Source: CAD feature listing. Evaluate the final solid. Frame: model axes, mm. A direction names the side the tool comes from. Coordinates: 2 decimals unless noted, no trailing zeros. Order: outer loops, then holes, each group sorted by start corner. A loop starts at its lowest first (then second) coordinate and runs counter-clockwise, first axis right, second up. Notation, with made-up numbers: (-14.5, 47) -> (16.5, 47) arc R10 ccw to (16.5, 66) -> close; hole circle Ø4 at (-38.75, -11.75). An arc over 180 degrees is marked (long way). Write item = value, one per line. Start each with the question number.
Item 1: Ray query, line 1 along Y through (x, z) = (0, 3.5); line 2 along X through (y, z) = (15, 4.25); line 3 along Y through (x, z) = (-2.5, 5.2). Return the intervals inside material, ascending. Write a range as [from, to].
Item 2: Set-up query: faces 5 (the flat face through (3, -33, 2)), 6 (the flat face through (0, 21, 3)), 7 (the flat face through (3, -33, 4)), 8 (the flat face through (-2, -33, 3)). Return all of +Z, -Z, +X, -X, +Y, -Y with unobstructed straight access to the full face (end or side cutting, diameter ignored); none if empty.
Item 3: Contact query for flat-ended pins moving along their axis: pin 1 (4.5 mm diameter, centred on x = 0.5, y = -34, fed in from +Z); pin 2 (2 mm diameter, centred on x = -6, z = 3, fed in from -Y); pin 3 (3.5 mm diameter, centred on y = -34.5, z = 2.5, fed in from -X). Output: stop coordinate, or through.
Item 4: Section query A-A (x = -6.75). Output: boundary loops of the cut face in (y, z).
Item 5: Section query D-D (x = 0). Output: boundary loops of the cut face in (y, z).
Item 6: Section query C-C (z = 3.1). Output: boundary loops of the cut face in (x, y), then the cut area to 3 significant figures.
Item 7: Mould query, pull axis Y, two halves, no side actions, for faces 1 (the flat face through (0, -31.8, 1.5)), 2 (the flat face through (0, -21, 3)), 3 (the flat face through (0, 28, 3)), 4 (the flat face through (-10, 0, 3)). Classes: released by +Y, released by -Y, zero draft, split by the parting line, or undercut.
Item 8: Section query B-B (y = -33). Output: boundary loops of the cut face in (x, z), then the cut area to 3 significant figures.
```python
from build123d import *

# Parameters (mm, degrees)
SKETCH1_W           = 28
SKETCH1_H           = 56
SKETCH1_W_2         = 20
SKETCH1_H_2         = 42
BOSS_EXTRUDE1_DEPTH = 6
SKETCH2_W           = 4
SKETCH2_H           = 3
SKETCH2_W_2         = 1.5
SKETCH2_H_2         = 2
BOSS_EXTRUDE2_DEPTH = 10
SKETCH3_R           = 1
CUT_EXTRUDE1_DEPTH  = 10


with BuildPart() as part:
    # Sketch1 → Boss-Extrude1 (new body)
    with BuildSketch(Plane.XY):
        Rectangle(SKETCH1_W, SKETCH1_H)
        Rectangle(SKETCH1_W_2, SKETCH1_H_2, mode=Mode.SUBTRACT)
    extrude(amount=BOSS_EXTRUDE1_DEPTH)

    # Sketch2 → Boss-Extrude2 (add)
    with BuildSketch(Plane.XZ.offset(28)):
        with Locations((0, 3)):
            Rectangle(SKETCH2_W, SKETCH2_H)
        with Locations((2.75, 3)):
            Rectangle(SKETCH2_W_2, SKETCH2_H_2)
    extrude(amount=BOSS_EXTRUDE2_DEPTH)

    # Sketch3 → Cut-Extrude1 (cut)
    with BuildSketch(Plane.XY.offset(4.5)):
        with Locations((0, -33)):
            Circle(SKETCH3_R)
    extrude(amount=-CUT_EXTRUDE1_DEPTH, mode=Mode.SUBTRACT)


solid = part.part
```
Computed:
q1.line_1 = [-38, -34], [-32, -21], [21, 28]
q1.line_2 = [-14, -10], [10, 14]
q1.line_3 = [-28, -21], [21, 28]
q2.face_5 = -Z, +X, -Y
q2.face_6 = +Z, -Z
q2.face_7 = +Z, +X, -Y
q2.face_8 = +Z, -Z, -X, -Y
q3.pin_1 = 4.5
q3.pin_2 = -28
q3.pin_3 = -2
q4.outline = (-28, 0) -> (-21, 0) -> (-21, 6) -> (-28, 6) -> close; (21, 0) -> (28, 0) -> (28, 6) -> (21, 6) -> close
q5.outline = (-38, 1.5) -> (-34, 1.5) -> (-34, 4.5) -> (-38, 4.5) -> close; (-32, 1.5) -> (-28, 1.5) -> (-28, 0) -> (-21, 0) -> (-21, 6) -> (-28, 6) -> (-28, 4.5) -> (-32, 4.5) -> close; (21, 0) -> (28, 0) -> (28, 6) -> (21, 6) -> close
q6.outline = (-14, -28) -> (-2, -28) -> (-2, -38) -> (3.5, -38) -> (3.5, -28) -> (14, -28) -> (14, 28) -> (-14, 28) -> close; hole (-10, -21) -> (10, -21) -> (10, 21) -> (-10, 21) -> close; hole circle Ø2 at (0, -33)
q6.area = 780 mm^2
q7.face_1 = zero draft
q7.face_2 = undercut
q7.face_3 = released by +Y
q7.face_4 = undercut
q8.outline = (-2, 1.5) -> (-1, 1.5) -> (-1, 4.5) -> (-2, 4.5) -> close; (1, 1.5) -> (2, 1.5) -> (2, 2) -> (3.5, 2) -> (3.5, 4) -> (2, 4) -> (2, 4.5) -> (1, 4.5) -> close
q8.area = 9.00 mm^2
